Check sheet for the modelled part. Datum: model origin and axes. Units: mm. A direction names the side the tool comes from. Coordinates: 2 decimals unless noted, no trailing zeros. Write each loop counter-clockwise with the first axis right and the second up, starting at its lowest first coordinate (ties: lowest second). Pieces come first, ordered by that corner, then holes. Notation, with made-up numbers: M 75.5,79 L 103.5,79 A25 ccw 103.5,112 Z; hole C 74,59 d6. An arc over 180 degrees is marked long. Answer as CSV lines item,"result". Start each with the question number.
Q1. Mould release check, pull along X, two halves, no side actions. Record for faces 1 (the cylindrical face through (17.248, -11.972, 17.287)), 2 (the cylindrical face through (-17.119, 0.14, 16.975)), 3 (the flat face through (-17, 10, 10)): pulls with the +X half, pulls with the -X half, needs draft (parallel to the pull), parting line crosses it, or undercut.
Q2. Sectioned sample at B-B, the plane y = -0.25. Record the cut outline in (x, z).
Q3. Sectioned sample at C-C, the plane x = 13.5. Record the cut outline in (y, z).
Q4. Sectioned sample at D-D, the plane z = 12.5. Record the cut outline in (x, y).
Q5. Access from +Z, -Z, +X, -X, +Y, -Y to the whole of each face (thin tool, end or side, straight path). Record for faces 4 (the flat face through (10, -10, -17)), 5 (the cylindrical face through (-16.975, 0.14, -17.119)), 6 (the flat face through (-17, 10, -10)), 7 (the flat face through (17.21, 10, 17.1)), 8 (the flat face through (17.5, 0, 0)).
Q6. Sectioned sample at A-A, the plane z = 5. Record the cut outline in (x, y).
Q7. Thickness scan on line 1 along X through (y, z) = (-11.5, 1); line 2 along Z through (x, y) = (14.75, 5.5). Record the ranges inside material, lowest first. Write a range as from..to.
Q8. Depth check by flat-ended pin: pin 1 Ø1 at (x, y) = (10, -5.5) entering from +Z. Enter the tip coordinate at first touch or a pass-through.
from build123d import *

# Parameters (mm, degrees)
F0_W     = 36
F0_H     = 36
F0_R     = 1.75
F1_DEPTH = 14
F3_DEPTH = 10
F4_R     = 2.5


with BuildPart() as f1:
    # F0 (on Front) → F1 (new body, symmetric)
    with BuildSketch(Plane.XZ):
        Rectangle(F0_W, F0_H)
        with Locations((-14.75, -14.75)):
            Circle(F0_R, mode=Mode.SUBTRACT)
        with Locations((14.75, -14.75)):
            Circle(F0_R, mode=Mode.SUBTRACT)
        with Locations((-14.75, 14.75)):
            Circle(F0_R, mode=Mode.SUBTRACT)
        with BuildLine():
            ThreePointArc((-17.5, 5.6841885964), (-13.0107647738, 13.0107647738), (-5.6841885964, 17.5))
            Line((-5.6841885964, 17.5), (5.6841885964, 17.5))
            ThreePointArc((5.6841885964, 17.5), (13.0107647738, 13.0107647738), (17.5, 5.6841885964))
            Line((17.5, 5.6841885964), (17.5, -5.6841885964))
            ThreePointArc((17.5, -5.6841885964), (13.0107647738, -13.0107647738), (5.6841885964, -17.5))
            Line((5.6841885964, -17.5), (-5.6841885964, -17.5))
            ThreePointArc((-5.6841885964, -17.5), (-13.0107647738, -13.0107647738), (-17.5, -5.6841885964))
            Line((-17.5, -5.6841885964), (-17.5, 5.6841885964))
        make_face(mode=Mode.SUBTRACT)
        with Locations((14.75, 14.75)):
            Circle(F0_R, mode=Mode.SUBTRACT)
    extrude(amount=F1_DEPTH, both=True)

    # F2 (on Front) → F3 (cut, symmetric)
    with BuildSketch(Plane.XZ):
        with BuildLine():
            ThreePointArc((-15.1093137054, 11.5199235828), (-17.0480970389, 17.0480970389), (-11.5199235828, 15.1093137054))
            ThreePointArc((-11.5199235828, 15.1093137054), (-8.9192295863, 16.7763924485), (-6.0827625303, 18))
            Line((-6.0827625303, 18), (-6.0827625303, 19))
            Line((-6.0827625303, 19), (-19, 19))
            Line((-19, 19), (-19, 6.0827625303))
            Line((-19, 6.0827625303), (-18, 6.0827625303))
            ThreePointArc((-18, 6.0827625303), (-16.7763924485, 8.9192295863), (-15.1093137054, 11.5199235828))
        make_face()
        with BuildLine():
            Line((19, 6.0827625303), (19, 19))
            Line((19, 19), (6.0827625303, 19))
            Line((6.0827625303, 19), (6.0827625303, 18))
            ThreePointArc((6.0827625303, 18), (8.9192295863, 16.7763924485), (11.5199235828, 15.1093137054))
            ThreePointArc((11.5199235828, 15.1093137054), (17.0480970389, 17.0480970389), (15.1093137054, 11.5199235828))
            ThreePointArc((15.1093137054, 11.5199235828), (16.7763924485, 8.9192295863), (18, 6.0827625303))
            Line((18, 6.0827625303), (19, 6.0827625303))
        make_face()
        with BuildLine():
            Line((-19, -6.0827625303), (-19, -19))
            Line((-19, -19), (-6.0827625303, -19))
            Line((-6.0827625303, -19), (-6.0827625303, -18))
            ThreePointArc((-6.0827625303, -18), (-8.9192295863, -16.7763924485), (-11.5199235828, -15.1093137054))
            ThreePointArc((-11.5199235828, -15.1093137054), (-17.0480970389, -17.0480970389), (-15.1093137054, -11.5199235828))
            ThreePointArc((-15.1093137054, -11.5199235828), (-16.7763924485, -8.9192295863), (-18, -6.0827625303))
            Line((-18, -6.0827625303), (-19, -6.0827625303))
        make_face()
        with BuildLine():
            Line((6.0827625303, -19), (19, -19))
            Line((19, -19), (19, -6.0827625303))
            Line((19, -6.0827625303), (18, -6.0827625303))
            ThreePointArc((18, -6.0827625303), (16.7763924485, -8.9192295863), (15.1093137054, -11.5199235828))
            ThreePointArc((15.1093137054, -11.5199235828), (17.0480970389, -17.0480970389), (11.5199235828, -15.1093137054))
            ThreePointArc((11.5199235828, -15.1093137054), (8.9192295863, -16.7763924485), (6.0827625303, -18))
            Line((6.0827625303, -18), (6.0827625303, -19))
        make_face()
    extrude(amount=F3_DEPTH, both=True, mode=Mode.SUBTRACT)

    # F4
    f4_edges = [f1.edges().sort_by_distance(p)[0] for p in [
        (18, -12, 18),
        (18, 12, 18),
        (18, -12, -18),
        (18, 12, -18),
        (-18, -12, 18),
        (-18, 12, 18),
        (-18, 12, -18),
        (-18, -12, -18),
    ]]
    fillet(f4_edges, radius=F4_R)


solid = f1.part
Output:
1,face 1,"pulls with the +X half"
1,face 2,"undercut"
1,face 3,"needs draft"
2,outline,"M -18,-6.08 A19 ccw -15.11,-11.52 A3.25 ccw long -11.52,-15.11 A19 ccw -6.08,-18 L 6.08,-18 A19 ccw 11.52,-15.11 A3.25 ccw long 15.11,-11.52 A19 ccw 18,-6.08 L 18,6.08 A19 ccw 15.11,11.52 A3.25 ccw long 11.52,15.11 A19 ccw 6.08,18 L -6.08,18 A19 ccw -11.52,15.11 A3.25 ccw long -15.11,11.52 A19 ccw -18,6.08 Z; hole M -17.5,-5.68 A18.4 ccw -5.68,-17.5 L 5.68,-17.5 A18.4 ccw 17.5,-5.68 L 17.5,5.68 A18.4 ccw 5.68,17.5 L -5.68,17.5 A18.4 ccw -17.5,5.68 Z; hole C -14.75,-14.75 d3.5; hole C -14.75,14.75 d3.5; hole C 14.75,-14.75 d3.5; hole C 14.75,14.75 d3.5"
3,outline,"M -14,-18 L -10,-18 L -10,-17.75 L 10,-17.75 L 10,-18 L 14,-18 L 14,-15.97 L -14,-15.97 Z; M -14,-13.53 L 14,-13.53 L 14,-12.5 L -14,-12.5 Z; M -14,12.5 L 14,12.5 L 14,13.53 L -14,13.53 Z; M -14,15.97 L 14,15.97 L 14,18 L 10,18 L 10,17.75 L -10,17.75 L -10,18 L -14,18 Z"
4,outline,"M -18,-14 L -13.5,-14 L -13.5,14 L -18,14 L -18,10 L -17.1,10 L -17.1,-10 L -18,-10 Z; M 13.5,-14 L 18,-14 L 18,-10 L 17.1,-10 L 17.1,10 L 18,10 L 18,14 L 13.5,14 Z"
5,face 4,"-Z"
5,face 5,"none"
5,face 6,"-X"
5,face 7,"+Z, +X"
5,face 8,"+Y, -Y"
6,outline,"M -18,-14 L -17.5,-14 L -17.5,14 L -18,14 Z; M 17.5,-14 L 18,-14 L 18,14 L 17.5,14 Z"
7,line 1,"x = -18..-17.5, 17.5..18"
7,line 2,"z = -18..-16.5, -13..-11, 11..13, 16.5..18"
8,pin 1,"stops at z = 16.45"
